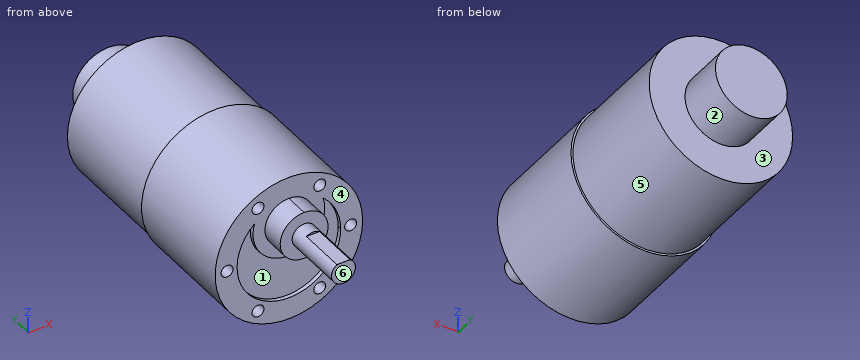
from build123d import *

# Parameters (mm, degrees)
F0_R      = 18.5
F0_R_2    = 18
F0_R_3    = 1.5
F0_R_4    = 3
F1_DEPTH  = 29
F2_R      = 18
F3_DEPTH  = 30
F4_R      = 9
F5_DEPTH  = 12
F6_DEPTH  = 6
F7_DEPTH  = 21.5
F8_DEPTH  = 10
F10_DEPTH = 12
F11_DEPTH = 1


with BuildPart() as f1:
    # F0 (on Front) → F1 (new body)
    with BuildSketch(Plane.XZ):
        Circle(F0_R)
        Circle(F0_R_2, mode=Mode.SUBTRACT)
        Circle(F0_R_2)
        with Locations((-7.75, -13.4233937587)):
            Circle(F0_R_3, mode=Mode.SUBTRACT)
        with Locations((7.75, -13.4233937587)):
            Circle(F0_R_3, mode=Mode.SUBTRACT)
        with Locations((-15.5, 0)):
            Circle(F0_R_3, mode=Mode.SUBTRACT)
        with Locations((-7.75, 13.4233937587)):
            Circle(F0_R_3, mode=Mode.SUBTRACT)
        with BuildLine():
            ThreePointArc((-8.5580252347, 9.7857142857), (-4.5708705218, 12.1699278007), (-4.3e-08, 13))
            ThreePointArc((-4.3e-08, 13), (4.5708704815, 12.1699278158), (8.5580252347, 9.7857142857))
            ThreePointArc((8.5580252347, 9.7857142857), (11.8375320074, 5.3733449521), (13, 0))
            ThreePointArc((13, 0), (-5.3733449521, -11.8375320074), (-8.5580252347, 9.7857142857))
        make_face(mode=Mode.SUBTRACT)
        with Locations((15.5, 0)):
            Circle(F0_R_3, mode=Mode.SUBTRACT)
        with Locations((7.75, 13.4233937587)):
            Circle(F0_R_3, mode=Mode.SUBTRACT)
        with BuildLine():
            ThreePointArc((13, 0), (11.8375320074, 5.3733449521), (8.5580252347, 9.7857142857))
            ThreePointArc((8.5580252347, 9.7857142857), (0, -2), (-8.5580252347, 9.7857142857))
            ThreePointArc((-8.5580252347, 9.7857142857), (-5.3733449521, -11.8375320074), (13, 0))
        make_face()
        with BuildLine():
            ThreePointArc((8.5580252347, 9.7857142857), (4.5708704815, 12.1699278158), (-4.3e-08, 13))
            ThreePointArc((-4.3e-08, 13), (-4.5708705218, 12.1699278007), (-8.5580252347, 9.7857142857))
            ThreePointArc((-8.5580252347, 9.7857142857), (0, -2), (8.5580252347, 9.7857142857))
        make_face()
        with BuildLine():
            ThreePointArc((-4.3e-08, 13), (4.2426406719, 11.2426407023), (6, 7))
            ThreePointArc((6, 7), (-4.2426406719, 2.7573592977), (-4.3e-08, 13))
        make_face(mode=Mode.SUBTRACT)
        with BuildLine():
            ThreePointArc((-4.3e-08, 13), (-4.2426406719, 2.7573592977), (6, 7))
            ThreePointArc((6, 7), (4.2426406719, 11.2426407023), (-4.3e-08, 13))
        make_face()
        with Locations((0, 7)):
            Circle(F0_R_4, mode=Mode.SUBTRACT)
        with Locations((0, 7)):
            Circle(F0_R_4)
        with Locations((-15.5, 0)):
            Circle(F0_R_3)
        with Locations((7.75, -13.4233937587)):
            Circle(F0_R_3)
        with Locations((15.5, 0)):
            Circle(F0_R_3)
        with Locations((7.75, 13.4233937587)):
            Circle(F0_R_3)
        with Locations((-7.75, -13.4233937587)):
            Circle(F0_R_3)
        with Locations((-7.75, 13.4233937587)):
            Circle(F0_R_3)
    extrude(amount=-F1_DEPTH)

    # F2 (on face) → F3 (join)
    with BuildSketch(Plane(origin=(0, 29, 0), x_dir=(-1, 0, 0), z_dir=(0, 1, 0))):
        Circle(F2_R)
    extrude(amount=F3_DEPTH)

    # F4 (on face) → F5 (join)
    with BuildSketch(Plane(origin=(0, 59, 0), x_dir=(-1, 0, 0), z_dir=(0, 1, 0))):
        Circle(F4_R)
    extrude(amount=F5_DEPTH)

    # F0 (on Front) → F6 (join)
    with BuildSketch(Plane.XZ):
        with BuildLine():
            ThreePointArc((-4.3e-08, 13), (-4.2426406719, 2.7573592977), (6, 7))
            ThreePointArc((6, 7), (4.2426406719, 11.2426407023), (-4.3e-08, 13))
        make_face()
        with Locations((0, 7)):
            Circle(F0_R_4, mode=Mode.SUBTRACT)
    extrude(amount=F6_DEPTH)

    # F0 (on Front) → F7 (join)
    with BuildSketch(Plane.XZ):
        with Locations((0, 7)):
            Circle(F0_R_4)
    extrude(amount=F7_DEPTH)

    # F0 (on Front) → F8 (cut)
    with BuildSketch(Plane.XZ):
        with Locations((-7.75, 13.4233937587)):
            Circle(F0_R_3)
        with Locations((7.75, 13.4233937587)):
            Circle(F0_R_3)
        with Locations((15.5, 0)):
            Circle(F0_R_3)
        with Locations((-7.75, -13.4233937587)):
            Circle(F0_R_3)
        with Locations((-15.5, 0)):
            Circle(F0_R_3)
        with Locations((7.75, -13.4233937587)):
            Circle(F0_R_3)
    extrude(amount=-F8_DEPTH, mode=Mode.SUBTRACT)

    # F9 (on face) → F10 (cut)
    with BuildSketch(Plane.XZ.offset(21.5)):
        with BuildLine():
            ThreePointArc((-1.6583123952, 9.5), (0, 10), (1.6583123952, 9.5))
            Line((1.6583123952, 9.5), (6.0122050345, 9.5))
            Line((6.0122050345, 9.5), (6.0122050345, 13.4357631467))
            Line((6.0122050345, 13.4357631467), (-7.3503456078, 13.4357631467))
            Line((-7.3503456078, 13.4357631467), (-7.3503456078, 9.5))
            Line((-7.3503456078, 9.5), (-1.6583123952, 9.5))
        make_face()
        with BuildLine():
            Line((-1.6583123952, 9.5), (1.6583123952, 9.5))
            ThreePointArc((1.6583123952, 9.5), (0, 10), (-1.6583123952, 9.5))
        make_face()
    extrude(amount=-F10_DEPTH, mode=Mode.SUBTRACT)

    # F0 (on Front) → F11 (cut)
    with BuildSketch(Plane.XZ):
        with BuildLine():
            ThreePointArc((13, 0), (11.8375320074, 5.3733449521), (8.5580252347, 9.7857142857))
            ThreePointArc((8.5580252347, 9.7857142857), (0, -2), (-8.5580252347, 9.7857142857))
            ThreePointArc((-8.5580252347, 9.7857142857), (-5.3733449521, -11.8375320074), (13, 0))
        make_face()
    extrude(amount=-F11_DEPTH, mode=Mode.SUBTRACT)


solid = f1.part
Model file for the job. Use its own axes, mm. Face numbers are marked on the shaded views. A direction names the side the tool comes from. Give positions to 0.01 mm unless a question says otherwise; leave off trailing zeros. Loops run counter-clockwise (first coordinate to the right, second up) from the corner with the lowest first, then second, coordinate; pieces in that order, holes last. Notation, with made-up numbers: (45, 62.5) -> (89, 62.5) arc R9 ccw to (89, 79.5) -> close; hole circle Ø6 at (89.25, -28). An arc over 180 degrees is marked (long way). Use a Markdown table: item, result. Add a question column.
(1) Drop flat-ended pins along their axis: pin 1 Ø3.5 at (x, z) = (7, -13.5) entering from -Y; pin 2 Ø1.8 at (x, z) = (15.5, 0) entering from +Y; pin 3 Ø1.8 at (x, z) = (7.75, -13.42) entering from -Y. Give the stop position or say it passes through.
(2) Tool access for the marked faces 4, 5 and 6: list every direction of +Z, -Z, +X, -X, +Y, -Y with a clear straight run to the whole face (end or side of a thin tool).
(3) Slice it at B-B on y = 6. List the corners of the cut face in (x, z), and give its area (3 significant figures).
(4) Mould opens along Z. For the marked faces 1, 2 and 3 say: +Z half, -Z half, draft (parallel to the pull), parting line (faces both ways), or undercut.
(5) Wall check: line 1 along Y through (x, z) = (-1, -17); line 2 along Z through (x, y) = (-7.75, 4.5); line 3 along Y through (x, z) = (12, 3). Give the ranges that are in metal, low to high.
(6) Slice it at D-D on y = -13.5. List the corners of the cut face in (x, z), and give its area (3 significant figures).
(7) Slice it at A-A on z = 8. List the corners of the cut face in (x, y), and give its area (3 significant figures).
(8) Slice it at C-C on x = 15. List the corners of the cut face in (y, z), and give its area (3 significant figures).
Filled sheet:
| question | item | result |
|---|---|---|
| 1 | pin 1 | y = 0 |
| 1 | pin 2 | y = 59 |
| 1 | pin 3 | y = 10 |
| 2 | face 4 | -Y |
| 2 | face 5 | +Y |
| 2 | face 6 | +Z, -Z, +X, -X, -Y |
| 3 | outline | circle Ø37 at (0, 0); hole circle Ø3 at (-15.5, 0); hole circle Ø3 at (-7.75, -13.42); hole circle Ø3 at (-7.75, 13.42); hole circle Ø3 at (7.75, -13.42); hole circle Ø3 at (7.75, 13.42); hole circle Ø3 at (15.5, 0) |
| 3 | area | 1,030 mm2 |
| 4 | face 1 | undercut |
| 4 | face 2 | parting line |
| 4 | face 3 | draft |
| 5 | line 1 | 0 to 59 |
| 5 | line 2 | -16.8 to -14.92, -11.92 to 11.92, 14.92 to 16.8 |
| 5 | line 3 | 1 to 59 |
| 6 | outline | (-1.66, 9.5) arc R3 ccw (long way) to (1.66, 9.5) -> close |
| 6 | area | 27.1 mm2 |
| 7 | outline | (-16.68, 0) -> (-10.25, 0) -> (-10.25, 1) -> (-8.94, 1) -> (-8.94, 0) -> (-5.92, 0) -> (-5.92, -6) -> (-2.83, -6) -> (-2.83, -21.5) -> (2.83, -21.5) -> (2.83, -6) -> (5.92, -6) -> (5.92, 0) -> (8.94, 0) -> (8.94, 1) -> (10.25, 1) -> (10.25, 0) -> (16.68, 0) -> (16.68, 29) -> (16.12, 29) -> (16.12, 59) -> (4.12, 59) -> (4.12, 71) -> (-4.12, 71) -> (-4.12, 59) -> (-16.12, 59) -> (-16.12, 29) -> (-16.68, 29) -> close |
| 7 | area | 2,190 mm2 |
| 8 | outline | (0, -10.83) -> (29, -10.83) -> (29, -9.95) -> (59, -9.95) -> (59, 9.95) -> (29, 9.95) -> (29, 10.83) -> (0, 10.83) -> (0, 1.41) -> (10, 1.41) -> (10, -1.41) -> (0, -1.41) -> close |
| 8 | area | 1,200 mm2 |
